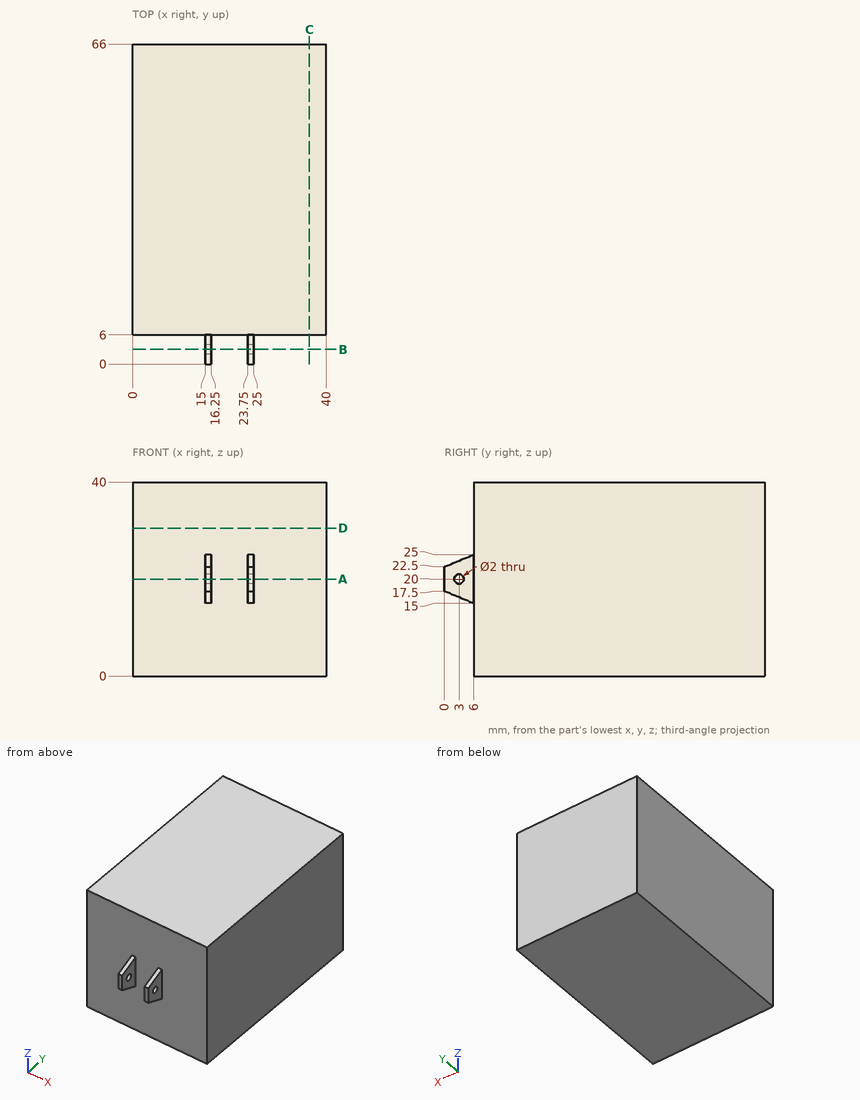
Drawing for the job (mm, zero at the part's lowest x, y, z). Round coordinates to 2 decimals unless told otherwise and drop trailing zeros. Write each loop counter-clockwise with the first axis right and the second up, starting at its lowest first coordinate (ties: lowest second). Pieces come first, ordered by that corner, then holes. Notation, with made-up numbers: (27, 61.25) - (51, 61.25) arc R7 cw to (51, 66.25) - close; hole circle Ø8 at (-22, -3). An arc over 180 degrees is marked (long way). Return JSON: item names as keys, results as strings. Group by question number.
Item 1: Band-saw the part on D-D on z = 30.5. List the corners of the cut face in (x, y), plus the area to 3 significant figures.
Item 2: Band-saw the part on B-B on y = 3. List the corners of the cut face in (x, z), plus the area to 4 significant figures.
Item 3: Band-saw the part on A-A on z = 20. List the corners of the cut face in (x, y).
Item 4: Probe probe 1 along Z at (x, y) = (15.3, 3); probe 2 along Y at (x, z) = (15.3, 20); probe 3 along Y at (x, z) = (35, 28). List the from-to ranges inside material, lowest first.
Item 5: Flat gauge pins, fed straight in: pin 1 Ø5 at (x, z) = (24.5, 31.5) entering from -Y; pin 2 Ø3 at (y, z) = (3, 21.5) entering from +X; pin 3 Ø1.8 at (y, z) = (2.5, 20) entering from -X. Where does each tip first touch, or does it go through?
Item 6: Band-saw the part on C-C on x = 36.5. List the corners of the cut face in (y, z).
Resolved:
{
 "1": {"outline": "(0, 6) - (40, 6) - (40, 66) - (0, 66) - close", "area": "2,400 mm²"},
 "2": {"outline": "(15, 16.25) - (16.25, 16.25) - (16.25, 19) - (15, 19) - close; (15, 21) - (16.25, 21) - (16.25, 23.75) - (15, 23.75) - close; (23.75, 16.25) - (25, 16.25) - (25, 19) - (23.75, 19) - close; (23.75, 21) - (25, 21) - (25, 23.75) - (23.75, 23.75) - close", "area": "13.75 mm²"},
 "3": {"outline": "(0, 6) - (15, 6) - (15, 4) - (16.25, 4) - (16.25, 6) - (23.75, 6) - (23.75, 4) - (25, 4) - (25, 6) - (40, 6) - (40, 66) - (0, 66) - close; (15, 0) - (16.25, 0) - (16.25, 2) - (15, 2) - close; (23.75, 0) - (25, 0) - (25, 2) - (23.75, 2) - close"},
 "4": {"probe 1": "z = 16.25 to 19, 21 to 23.75", "probe 2": "y = 0 to 2, 4 to 66", "probe 3": "y = 6 to 66"},
 "5": {"pin 1": "stops at y = 6", "pin 2": "stops at x = 25", "pin 3": "stops at x = 15"},
 "6": {"outline": "(6, 0) - (66, 0) - (66, 40) - (6, 40) - close"}
}
